Geometry: final body of the model. Coordinates: model frame, mm. A direction names the side the tool comes from. Give positions to 0.01 mm unless a question says otherwise; leave off trailing zeros. Write each loop counter-clockwise with the first axis right and the second up, starting at its lowest first coordinate (ties: lowest second). Pieces come first, ordered by that corner, then holes. Notation, with made-up numbers: (-15, 76.25) -> (25, 76.25) arc R34 cw to (25, 115.25) -> close; hole circle Ø9 at (37, 30). An arc over 180 degrees is marked (long way). Answer in a Markdown table with one row per item. Add a question column.
from build123d import *

# Parameters (mm, degrees)
EXTRUDE_THIN1_DEPTH       = 80
BOSS_EXTRUDE1_START       = -10
BOSS_EXTRUDE1_DEPTH       = 10
SKETCH3_R                 = 2.25
BOSS_EXTRUDE2_DEPTH       = 5
BOSS_EXTRUDE3_DEPTH       = 10
SKETCH5_R                 = 2.25
CUT_EXTRUDE1_DEPTH        = 6
BOSS_EXTRUDE4_REACH       = 104.415
BOSS_EXTRUDE4_END_RADIUS  = 39
SKETCH10_W                = 20
SKETCH10_H                = 20
BOSS_EXTRUDE6_DEPTH       = 6
BOSS_EXTRUDE7_START       = -51.724499634
BOSS_EXTRUDE7_OUTLINE_W   = 20
BOSS_EXTRUDE7_OUTLINE_H   = 20
BOSS_EXTRUDE7_DEPTH       = 51.724499634
BOSS_EXTRUDE7_START_2     = 101.306507824
BOSS_EXTRUDE7_2_OUTLINE_W = 23
BOSS_EXTRUDE7_2_OUTLINE_H = 23
BOSS_EXTRUDE7_2_DEPTH     = 3.693492176
BOSS_EXTRUDE9_DEPTH       = 20
SKETCH16_R                = 2.5
CUT_EXTRUDE2_DEPTH        = 20


with BuildPart() as part:
    # Sketch1 → Extrude-Thin1 (new body)
    with BuildSketch(Plane.XY):
        with BuildLine():
            ThreePointArc((-35, 0), (0, -35), (35, 0))
            Line((35, 0), (39, 0))
            ThreePointArc((39, 0), (0, -39), (-39, 0))
            Line((-39, 0), (-35, 0))
        make_face()
    extrude(amount=EXTRUDE_THIN1_DEPTH)

    # Sketch2 → Boss-Extrude1 (add)
    with BuildSketch(Plane.XY.offset(80).offset(BOSS_EXTRUDE1_START)):
        with BuildLine():
            Line((0, -39), (0, -35))
            Line((0, -35), (-10, -35))
            Line((-10, -35), (-10, -37.69615365))
            ThreePointArc((-10, -37.69615365), (-5.042321274, -38.672664715), (0, -39))
        make_face()
        with BuildLine():
            Line((10, -35), (0, -35))
            Line((0, -35), (0, -39))
            ThreePointArc((0, -39), (5.042321274, -38.672664715), (10, -37.69615365))
            Line((10, -37.69615365), (10, -35))
        make_face()
        with BuildLine():
            ThreePointArc((10, -37.69615365), (5.042321274, -38.672664715), (0, -39))
            ThreePointArc((0, -39), (-5.042321274, -38.672664715), (-10, -37.69615365))
            Line((-10, -37.69615365), (-10, -43))
            Line((-10, -43), (10, -43))
            Line((10, -43), (10, -37.69615365))
        make_face()
    extrude(amount=BOSS_EXTRUDE1_DEPTH)

    # Sketch3 → Boss-Extrude2 (add)
    with BuildSketch(Plane.XY.offset(80)):
        with Locations((-5, -39)):
            Circle(SKETCH3_R)
        with Locations((5, -39)):
            Circle(SKETCH3_R)
    extrude(amount=BOSS_EXTRUDE2_DEPTH)

    # Sketch4 → Boss-Extrude3 (add)
    with BuildSketch(Plane(origin=(0, 0, 0), x_dir=(-1, 0, 0), z_dir=(0, 0, -1))):
        with BuildLine():
            Line((0, -39), (0, -35))
            Line((0, -35), (-10, -35))
            Line((-10, -35), (-10, -37.69615365))
            ThreePointArc((-10, -37.69615365), (-5.042321274, -38.672664715), (0, -39))
        make_face()
        with BuildLine():
            ThreePointArc((10, -37.69615365), (5.042321274, -38.672664715), (0, -39))
            ThreePointArc((0, -39), (-5.042321274, -38.672664715), (-10, -37.69615365))
            Line((-10, -37.69615365), (-10, -43))
            Line((-10, -43), (10, -43))
            Line((10, -43), (10, -37.69615365))
        make_face()
        with BuildLine():
            Line((10, -35), (0, -35))
            Line((0, -35), (0, -39))
            ThreePointArc((0, -39), (5.042321274, -38.672664715), (10, -37.69615365))
            Line((10, -37.69615365), (10, -35))
        make_face()
    extrude(amount=-BOSS_EXTRUDE3_DEPTH)

    # Sketch5 → Cut-Extrude1 (cut)
    with BuildSketch(Plane(origin=(0, 0, 0), x_dir=(-1, 0, 0), z_dir=(0, 0, -1))):
        with Locations(Location((-5, -39, 0), (0, 0, 180))):
            Circle(SKETCH5_R)
        with Locations(Location((5, -39, 0), (0, 0, 180))):
            Circle(SKETCH5_R)
    extrude(amount=-CUT_EXTRUDE1_DEPTH, mode=Mode.SUBTRACT)

    # Boss-Extrude4: up to this cylinder (the profile starts outside it)
    boss_extrude4_end = Plane(origin=(0, 0, 40), z_dir=(0, 0, -1)) * Cylinder(BOSS_EXTRUDE4_END_RADIUS, 287.83, mode=Mode.PRIVATE)
    # Sketch10 → Boss-Extrude4 (add, up to the surface)
    with BuildSketch(Plane(origin=(0, -49.619293796, 4.341125699), x_dir=(1, 0, 0), z_dir=(0, 0.9961946980917462, -0.08715574274765152)), mode=Mode.PRIVATE) as boss_extrude4_sk1:
        with Locations((0, -35.795085407)):
            Rectangle(SKETCH10_W, SKETCH10_H)
    boss_extrude4_tool1 = extrude(boss_extrude4_sk1.sketch, amount=BOSS_EXTRUDE4_REACH, mode=Mode.PRIVATE) - boss_extrude4_end
    add(boss_extrude4_tool1.solids().sort_by_distance((0, -46.499547, 40))[0])

    # Sketch14 → Boss-Extrude6 (add)
    with BuildSketch(Plane(origin=(0, -0.732594735, -5.56460947), x_dir=(1, 0, 0), z_dir=(0, 0.130526192220045, 0.9914448613738114))):
        with BuildLine():
            Line((-39, 0), (-39, 50))
            Line((-39, 50), (39, 50))
            Line((39, 50), (39, 0))
            ThreePointArc((39, 0), (0, -39), (-39, 0))
        make_face()
    extrude(amount=BOSS_EXTRUDE6_DEPTH)

    # Boss-Extrude7: read off the stored shape, not the designer's step
    # Boss-Extrude7 outline → Boss-Extrude7 (add)
    with BuildSketch(Plane(origin=(0, -49.619293796, 4.341125699), x_dir=(1, 0, 0), z_dir=(0, 0.9961946980917462, -0.08715574274765152)).offset(BOSS_EXTRUDE7_START)):
        with Locations((0, -35.795085407)):
            Rectangle(BOSS_EXTRUDE7_OUTLINE_W, BOSS_EXTRUDE7_OUTLINE_H)
    extrude(amount=BOSS_EXTRUDE7_DEPTH)

    # Boss-Extrude7 2 outline → Boss-Extrude7 2 (cut)
    with BuildSketch(Plane(origin=(0, 0, 0), x_dir=(0.9966522374056315, 0.08110432407614718, -0.010315342480997143), z_dir=(0.08175767654690885, -0.9886876617314986, 0.1257473254807149)).offset(BOSS_EXTRUDE7_START_2)):
        with Locations((-8.5, 31.5)):
            Rectangle(BOSS_EXTRUDE7_2_OUTLINE_W, BOSS_EXTRUDE7_2_OUTLINE_H)
    extrude(amount=BOSS_EXTRUDE7_2_DEPTH, mode=Mode.SUBTRACT)

    # Sketch15 → Boss-Extrude9 (add, along a direction that is not the sketch's normal)
    with BuildSketch(Plane(origin=(10, 0, 0), x_dir=(0, 0, -1), z_dir=(1, 0, 0))):
        Polygon((-54.258496601, -94.737775996), (-34.403038319, -97.263114251), (-33.528151684, -87.263114251), (-53.383609966, -84.737775996), align=None)
    extrude(amount=BOSS_EXTRUDE9_DEPTH, dir=(0.9966471031139099, 0.08150889038643343, -0.007131103885357661))

    # Sketch16 → Cut-Extrude2 (cut)
    with BuildSketch(Plane(origin=(7.465262096, -90.276691283, 11.481940072), x_dir=(0.9966522374056315, 0.08110432407614722, -0.010315342480997126), z_dir=(-0.0817576765469089, 0.9886876617314987, -0.12574732548071466))):
        with Locations(Location((12.543149078, -37.29773566, 0), (0, 0, 270))):
            Circle(SKETCH16_R)
        with Locations(Location((12.543149078, -27.282379188, 0), (0, 0, 270))):
            Circle(SKETCH16_R)
    extrude(amount=-CUT_EXTRUDE2_DEPTH, mode=Mode.SUBTRACT)


solid = part.part
Q1. Section D-D on x = 5. Return loops of the section in (y, z).
Q2. Section B-B on x = -5. Return loops of the section in (y, z).
Q3. Section A-A on x = 15. Return loops of the section in (y, z), and give its area (3 significant figures).
Q4. Contact query for flat-ended pins moving along their axis: pin 1 Ø2 at (x, z) = (-4.5, 60.5) entering from +Y; pin 2 Ø12 at (x, y) = (-9, -29) entering from -Z; pin 3 Ø7.5 at (y, z) = (-72, 47.5) entering from -X. Output: stop coordinate, or through.
Q5. Line query: probe 1 along X at (y, z) = (-39, 3); probe 2 along Z at (x, y) = (25, 10); probe 3 along Z at (x, y) = (-19, 3). Output: solid intervals per line, ascending. Write a range as from..to.
Q6. Pull-direction query (Y, two-part tool) for faces 1 (the cylindrical face through (4.71, -36.77, 82.46)), 2 (the flat face through (19.827, -85.214, 43.247)), 3 (the flat face through (-39, 24, -6)), 4 (the flat face through (37, 0, 39)); classes: +Y half, -Y half, draft (parallel to the pull), parting line (faces both ways), or undercut.
Q7. Access query for faces 5 (the cylindrical face through (18.16, -89.46, 50.14)), 6 (the flat face through (0.55, 7.9, -0.65)), 7 (the flat face through (0, -43, 5)), 8 (the flat face through (-10, -68, 42)). Directions: +Z, -Z, +X, -X, +Y, -Y. A direction counts if a zero-diameter tool reaches every point of the face in a straight line with its end or side. Return the directions, or none.
Q8. Section C-C on y = 39.5. Return loops of the section in (x, z).
Checks:
| question | item | result |
|---|---|---|
| 1 | outline | (-97.67, 34.44) -> (-38.68, 29.28) -> (-38.68, 10) -> (-43, 10) -> (-43, 0) -> (-41.25, 0) -> (-41.25, 6) -> (-36.75, 6) -> (-36.75, 5.23) -> (-38.3, 5.43) -> (-39.08, -0.52) -> (48.84, -12.09) -> (49.62, -6.14) -> (-34.64, 4.95) -> (-34.64, 80) -> (-36.75, 80) -> (-36.75, 85) -> (-41.25, 85) -> (-41.25, 80) -> (-43, 80) -> (-43, 70) -> (-38.68, 70) -> (-38.68, 49.35) -> (-95.15, 54.29) -> close |
| 2 | outline | (-98.49, 34.51) -> (-38.68, 29.28) -> (-38.68, 10) -> (-43, 10) -> (-43, 0) -> (-41.25, 0) -> (-41.25, 6) -> (-36.75, 6) -> (-36.75, 5.23) -> (-38.3, 5.43) -> (-39.08, -0.52) -> (48.84, -12.09) -> (49.62, -6.14) -> (-34.64, 4.95) -> (-34.64, 80) -> (-36.75, 80) -> (-36.75, 85) -> (-41.25, 85) -> (-41.25, 80) -> (-43, 80) -> (-43, 70) -> (-38.68, 70) -> (-38.68, 49.35) -> (-95.96, 54.37) -> close |
| 3 | outline | (-96.85, 34.37) -> (-86.85, 33.49) -> (-84.33, 53.35) -> (-94.33, 54.22) -> close; (-36.42, -0.87) -> (48.84, -12.09) -> (49.62, -6.14) -> (-31.62, 4.55) -> (-31.62, 80) -> (-36, 80) -> (-36, 2.36) -> close |
| 3 | area | 1,050 mm^2 |
| 4 | pin 1 | y = -34.57 |
| 4 | pin 2 | z = -2.63 |
| 4 | pin 3 | x = -10 |
| 5 | probe 1 | -10..-7.25, -2.75..2.75, 7.25..10 |
| 5 | probe 2 | -6.98..-0.93 |
| 5 | probe 3 | -6.06..0 |
| 6 | face 1 | parting line |
| 6 | face 2 | undercut |
| 6 | face 3 | draft |
| 6 | face 4 | +Y half |
| 7 | face 5 | none |
| 7 | face 6 | +Z, +Y |
| 7 | face 7 | -Z, +X, -X, -Y |
| 7 | face 8 | +Z, -Z, -X, -Y |
| 8 | outline | (-39, -10.86) -> (39, -10.86) -> (39, -4.81) -> (-39, -4.81) -> close |
